The listing builds one solid part. Answer for the finished solid, in the listing's coordinates (mm). Face numbers are marked on the shaded views. A direction names the side the tool comes from. Coordinates: 2 decimals unless noted, no trailing zeros. Loops run counter-clockwise (first coordinate to the right, second up) from the corner with the lowest first, then second, coordinate; pieces in that order, holes last. Notation, with made-up numbers: (30.25, 22.5) - (77.25, 22.5) arc R13 cw to (77.25, 44.5) - close; hole circle Ø7 at (37, 34.5). An arc over 180 degrees is marked (long way). Return JSON: item names as keys, results as strings. Group by question number.
1. Which of the six approach directions +Z, -Z, +X, -X, +Y, -Y give full straight-line access (tool end or side, diameter ignored) to the marked faces 4, 5 and 6?
2. Section C-C (x = -29) is taken. Write down the section's boundary in (y, z).
3. Find the intervals of material crossed by line 1 along Y through (x, z) = (-67, 19.5); line 2 along X through (y, z) = (13.5, 12.5); line 3 along Z through (x, y) = (-88, 10), in increasing order.
4. Section A-A (z = 6) is taken. Write down the section's boundary in (x, y).
5. Section D-D (z = 42) is taken. Write down the section's boundary in (x, y) (3 decimals), and give its area (3 significant figures).
6. Section B-B (y = 17) is taken. Write down the section's boundary in (x, z), and give its area (3 significant figures).
7. Each of these flat-tipped pins is pushed along its axis until it touches: P1, Ø10, axis at x = -36.5, y = 18.5, coming from the +Z side; P2, Ø8, axis at x = -17, y = 15, coming from the -Z side; P3, Ø7.5, axis at x = -92, z = 68, coming from the +Y side; P4, Ø1.9, axis at y = 3.5, z = 60.5, coming from the +X side (3 decimals). Where does it stop, or does it pass through?
8. The mould has two halves that part along X. Classify the marked faces 1, 2 and 3: pulls with the +X half, pulls with the -X half, needs draft (parallel to the pull), parting line crosses it, or undercut.
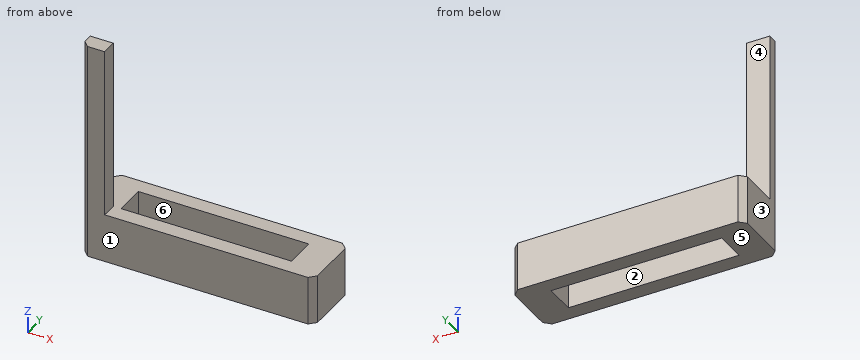
```python
from build123d import *

# Parameters (mm, degrees)
SKETCH1_W           = 95.25
SKETCH1_H           = 25.4
SKETCH1_W_2         = 69.85
SKETCH1_H_2         = 12.7
BOSS_EXTRUDE1_DEPTH = 20
SKETCH2_W           = 9.525
SKETCH2_H           = 6.35
BOSS_EXTRUDE2_DEPTH = 70
CHAMFER1_SIZE       = 2.54


with BuildPart() as part:
    # Sketch1 → Boss-Extrude1 (new body)
    with BuildSketch(Plane.XY):
        with Locations((-47.625, 12.7)):
            Rectangle(SKETCH1_W, SKETCH1_H)
        with Locations((-47.625, 12.7)):
            Rectangle(SKETCH1_W_2, SKETCH1_H_2, mode=Mode.SUBTRACT)
    extrude(amount=BOSS_EXTRUDE1_DEPTH)

    # Sketch2 → Boss-Extrude2 (add)
    with BuildSketch(Plane.XY.offset(20)):
        with Locations((-90.4875, 3.175)):
            Rectangle(SKETCH2_W, SKETCH2_H)
    extrude(amount=BOSS_EXTRUDE2_DEPTH)

    # Chamfer1
    chamfer1_edges = [part.edges().sort_by_distance(p)[0] for p in [
        (-95.25, 25.4, 10),
        (0, 25.4, 10),
        (0, 0, 10),
        (-95.25, 0, 45),
    ]]
    chamfer(chamfer1_edges, length=CHAMFER1_SIZE)


solid = part.part
```
The answers:
{
 "1": {"face 4": "+Z, +X, -X, +Y", "face 5": "-Z, +X, -X, +Y, -Y", "face 6": "+Z, -Z"},
 "2": {"outline": "(0, 0) - (6.35, 0) - (6.35, 20) - (0, 20) - close; (19.05, 0) - (25.4, 0) - (25.4, 20) - (19.05, 20) - close"},
 "3": {"line 1": "y = 0 to 6.35, 19.05 to 25.4", "line 2": "x = -95.25 to -82.55, -12.7 to 0", "line 3": "z = 0 to 20"},
 "4": {"outline": "(-95.25, 2.54) - (-92.71, 0) - (-2.54, 0) - (0, 2.54) - (0, 22.86) - (-2.54, 25.4) - (-92.71, 25.4) - (-95.25, 22.86) - close; hole (-82.55, 6.35) - (-12.7, 6.35) - (-12.7, 19.05) - (-82.55, 19.05) - close"},
 "5": {"outline": "(-95.25, 2.54) - (-92.71, 0) - (-85.725, 0) - (-85.725, 6.35) - (-95.25, 6.35) - close", "area": "57.3 mm2"},
 "6": {"outline": "(-95.25, 0) - (-82.55, 0) - (-82.55, 20) - (-95.25, 20) - close; (-12.7, 0) - (0, 0) - (0, 20) - (-12.7, 20) - close", "area": "508 mm2"},
 "7": {"P1": "stops at z = 20", "P2": "passes through", "P3": "stops at y = 6.35", "P4": "stops at x = -85.725"},
 "8": {"face 1": "needs draft", "face 2": "undercut", "face 3": "pulls with the -X half"}
}
